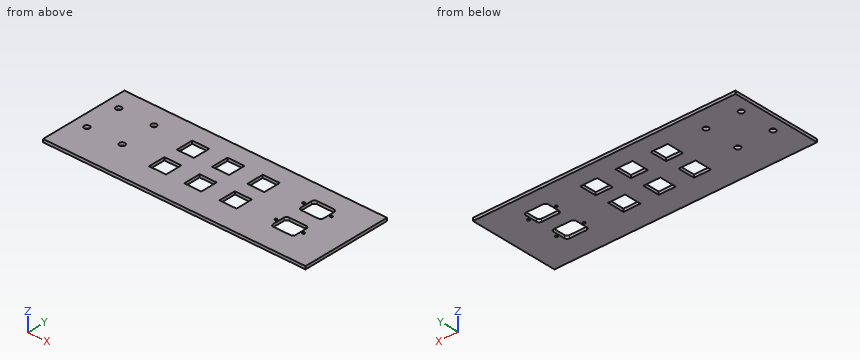
```python
from build123d import *

# Parameters (mm, degrees)
SKETCH1_W               = 378.46
SKETCH1_H               = 129.9972
BOSS_EXTRUDE1_DEPTH     = 4.191
F_3_8_16_TAPPED_HOLE1_D = 7.9375
CUT_EXTRUDE1_REACH      = 402.186
SKETCH5_W               = 24.5
SKETCH5_H               = 24.5
CUT_EXTRUDE2_REACH      = 402.186
SKETCH7_R               = 1.75


with BuildPart() as part:
    # Sketch1 → Boss-Extrude1 (new body)
    with BuildSketch(Plane.XY):
        with Locations((189.23, 64.9986)):
            Rectangle(SKETCH1_W, SKETCH1_H)
    extrude(amount=BOSS_EXTRUDE1_DEPTH)

    # 3/8-16 Tapped Hole1 (through all)
    with Locations(Plane.XY.offset(4.191)):
        with Locations((19.05, 99.8347), (69.85, 99.8347), (69.85, 49.0347), (19.05, 49.0347)):
            Hole(F_3_8_16_TAPPED_HOLE1_D / 2)

    # Sketch5 → Cut-Extrude1 (cut, up to next)
    with BuildSketch(Plane.XY.offset(4.191), mode=Mode.PRIVATE) as cut_extrude1_sk1:
        with Locations((132.9, 92.3472)):
            Rectangle(SKETCH5_W, SKETCH5_H)
    cut_extrude1_tool1 = extrude(cut_extrude1_sk1.sketch, amount=-CUT_EXTRUDE1_REACH, mode=Mode.PRIVATE) & part.part
    # Sketch5 → Cut-Extrude1 (cut, up to next)
    with BuildSketch(Plane.XY.offset(4.191), mode=Mode.PRIVATE) as cut_extrude1_sk2:
        with Locations((183.7, 92.3472)):
            Rectangle(SKETCH5_W, SKETCH5_H)
    cut_extrude1_tool2 = extrude(cut_extrude1_sk2.sketch, amount=-CUT_EXTRUDE1_REACH, mode=Mode.PRIVATE) & part.part
    # Sketch5 → Cut-Extrude1 (cut, up to next)
    with BuildSketch(Plane.XY.offset(4.191), mode=Mode.PRIVATE) as cut_extrude1_sk3:
        with Locations((234.5, 92.3472)):
            Rectangle(SKETCH5_W, SKETCH5_H)
    cut_extrude1_tool3 = extrude(cut_extrude1_sk3.sketch, amount=-CUT_EXTRUDE1_REACH, mode=Mode.PRIVATE) & part.part
    # Sketch5 → Cut-Extrude1 (cut, up to next)
    with BuildSketch(Plane.XY.offset(4.191), mode=Mode.PRIVATE) as cut_extrude1_sk4:
        with Locations((183.7, 47.8972)):
            Rectangle(SKETCH5_W, SKETCH5_H)
    cut_extrude1_tool4 = extrude(cut_extrude1_sk4.sketch, amount=-CUT_EXTRUDE1_REACH, mode=Mode.PRIVATE) & part.part
    # Sketch5 → Cut-Extrude1 (cut, up to next)
    with BuildSketch(Plane.XY.offset(4.191), mode=Mode.PRIVATE) as cut_extrude1_sk5:
        with Locations((234.5, 47.8972)):
            Rectangle(SKETCH5_W, SKETCH5_H)
    cut_extrude1_tool5 = extrude(cut_extrude1_sk5.sketch, amount=-CUT_EXTRUDE1_REACH, mode=Mode.PRIVATE) & part.part
    # Sketch5 → Cut-Extrude1 (cut, up to next)
    with BuildSketch(Plane.XY.offset(4.191), mode=Mode.PRIVATE) as cut_extrude1_sk6:
        with Locations((132.9, 47.8972)):
            Rectangle(SKETCH5_W, SKETCH5_H)
    cut_extrude1_tool6 = extrude(cut_extrude1_sk6.sketch, amount=-CUT_EXTRUDE1_REACH, mode=Mode.PRIVATE) & part.part
    add(cut_extrude1_tool1.solids().sort_by_distance((132.9, 92.3472, 4.191))[0], mode=Mode.SUBTRACT)
    add(cut_extrude1_tool2.solids().sort_by_distance((183.7, 92.3472, 4.191))[0], mode=Mode.SUBTRACT)
    add(cut_extrude1_tool3.solids().sort_by_distance((234.5, 92.3472, 4.191))[0], mode=Mode.SUBTRACT)
    add(cut_extrude1_tool4.solids().sort_by_distance((183.7, 47.8972, 4.191))[0], mode=Mode.SUBTRACT)
    add(cut_extrude1_tool5.solids().sort_by_distance((234.5, 47.8972, 4.191))[0], mode=Mode.SUBTRACT)
    add(cut_extrude1_tool6.solids().sort_by_distance((132.9, 47.8972, 4.191))[0], mode=Mode.SUBTRACT)

    # Sketch7 → Cut-Extrude2 (cut, up to next)
    with BuildSketch(Plane.XY.offset(4.191), mode=Mode.PRIVATE) as cut_extrude2_sk1:
        with Locations((292.657, 92.0972)):
            Circle(SKETCH7_R)
    cut_extrude2_tool1 = extrude(cut_extrude2_sk1.sketch, amount=-CUT_EXTRUDE2_REACH, mode=Mode.PRIVATE) & part.part
    # Sketch7 → Cut-Extrude2 (cut, up to next)
    with BuildSketch(Plane.XY.offset(4.191), mode=Mode.PRIVATE) as cut_extrude2_sk2:
        with Locations((332.657, 92.0972)):
            Circle(SKETCH7_R)
    cut_extrude2_tool2 = extrude(cut_extrude2_sk2.sketch, amount=-CUT_EXTRUDE2_REACH, mode=Mode.PRIVATE) & part.part
    # Sketch7 → Cut-Extrude2 (cut, up to next)
    with BuildSketch(Plane.XY.offset(4.191), mode=Mode.PRIVATE) as cut_extrude2_sk3:
        with Locations((332.657, 47.6472)):
            Circle(SKETCH7_R)
    cut_extrude2_tool3 = extrude(cut_extrude2_sk3.sketch, amount=-CUT_EXTRUDE2_REACH, mode=Mode.PRIVATE) & part.part
    # Sketch7 → Cut-Extrude2 (cut, up to next)
    with BuildSketch(Plane.XY.offset(4.191), mode=Mode.PRIVATE) as cut_extrude2_sk4:
        with Locations((292.657, 47.6472)):
            Circle(SKETCH7_R)
    cut_extrude2_tool4 = extrude(cut_extrude2_sk4.sketch, amount=-CUT_EXTRUDE2_REACH, mode=Mode.PRIVATE) & part.part
    # Sketch7 → Cut-Extrude2 (cut, up to next)
    with BuildSketch(Plane.XY.offset(4.191), mode=Mode.PRIVATE) as cut_extrude2_sk5:
        with BuildLine():
            Line((300.407, 60.1472), (324.907, 60.1472))
            ThreePointArc((324.907, 60.1472), (327.735427125, 58.975627125), (328.907, 56.1472))
            Line((328.907, 56.1472), (328.907, 39.1472))
            ThreePointArc((328.907, 39.1472), (327.735427125, 36.318772875), (324.907, 35.1472))
            Line((324.907, 35.1472), (300.407, 35.1472))
            ThreePointArc((300.407, 35.1472), (297.578572875, 36.318772875), (296.407, 39.1472))
            Line((296.407, 39.1472), (296.407, 56.1472))
            ThreePointArc((296.407, 56.1472), (297.578572875, 58.975627125), (300.407, 60.1472))
        make_face()
    cut_extrude2_tool5 = extrude(cut_extrude2_sk5.sketch, amount=-CUT_EXTRUDE2_REACH, mode=Mode.PRIVATE) & part.part
    # Sketch7 → Cut-Extrude2 (cut, up to next)
    with BuildSketch(Plane.XY.offset(4.191), mode=Mode.PRIVATE) as cut_extrude2_sk6:
        with BuildLine():
            Line((300.407, 104.5972), (324.907, 104.5972))
            ThreePointArc((324.907, 104.5972), (327.735427125, 103.425627125), (328.907, 100.5972))
            Line((328.907, 100.5972), (328.907, 83.5972))
            ThreePointArc((328.907, 83.5972), (327.735427125, 80.768772875), (324.907, 79.5972))
            Line((324.907, 79.5972), (300.407, 79.5972))
            ThreePointArc((300.407, 79.5972), (297.578572875, 80.768772875), (296.407, 83.5972))
            Line((296.407, 83.5972), (296.407, 100.5972))
            ThreePointArc((296.407, 100.5972), (297.578572875, 103.425627125), (300.407, 104.5972))
        make_face()
    cut_extrude2_tool6 = extrude(cut_extrude2_sk6.sketch, amount=-CUT_EXTRUDE2_REACH, mode=Mode.PRIVATE) & part.part
    add(cut_extrude2_tool1.solids().sort_by_distance((292.657, 92.0972, 4.191))[0], mode=Mode.SUBTRACT)
    add(cut_extrude2_tool2.solids().sort_by_distance((332.657, 92.0972, 4.191))[0], mode=Mode.SUBTRACT)
    add(cut_extrude2_tool3.solids().sort_by_distance((332.657, 47.6472, 4.191))[0], mode=Mode.SUBTRACT)
    add(cut_extrude2_tool4.solids().sort_by_distance((292.657, 47.6472, 4.191))[0], mode=Mode.SUBTRACT)
    add(cut_extrude2_tool5.solids().sort_by_distance((312.657, 47.6472, 4.191))[0], mode=Mode.SUBTRACT)
    add(cut_extrude2_tool6.solids().sort_by_distance((312.657, 92.0972, 4.191))[0], mode=Mode.SUBTRACT)


solid = part.part
```
Read the model definition and answer for the solid it produces. Units are mm, in the model's axes. Give positions to 0.01 mm unless a question says otherwise; leave off trailing zeros. Loops run counter-clockwise (first coordinate to the right, second up) from the corner with the lowest first, then second, coordinate; pieces in that order, holes last.
Item 1: The part is cut by section B-B (x = 140). Write down the section's boundary in (y, z), and give its area (3 significant figures).
Item 2: The part is cut by section C-C (z = 2.7). Give the number of separate pieces and of enclosed holes in the cut face, and give its area (3 significant figures).
Item 3: The part is cut by section A-A (x = 69.85). Write down the section's boundary in (y, z).
Item 4: Each of these flat-tipped pins is pushed along its axis until it touches: pin 1 Ø12.5 at (x, y) = (69.85, 49.03) entering from +Z; pin 2 Ø2 at (x, y) = (313.5, 102.5) entering from +Z. Where does it stop, or does it pass through?
Item 5: Find the intervals of material crossed by line 1 along Y through (x, z) = (245, 3); line 2 along X through (y, z) = (83, 2.9); line 3 along X through (y, z) = (42, 1.7), in increasing order.
Taken from the geometry:
1. outline: (0, 0) - (35.65, 0) - (35.65, 4.19) - (0, 4.19) - close; (60.15, 0) - (80.1, 0) - (80.1, 4.19) - (60.15, 4.19) - close; (104.6, 0) - (130, 0) - (130, 4.19) - (104.6, 4.19) - close
1. area: 339 mm2
2. separate pieces: 1
2. enclosed holes: 16
2. area: 43,800 mm2
3. outline: (0, 0) - (45.07, 0) - (45.07, 4.19) - (0, 4.19) - close; (53, 0) - (95.87, 0) - (95.87, 4.19) - (53, 4.19) - close; (103.8, 0) - (130, 0) - (130, 4.19) - (103.8, 4.19) - close
4. pin 1: stops at z = 4.19
4. pin 2: passes through
5. line 1: y = 0 to 35.65, 60.15 to 80.1, 104.6 to 130
5. line 2: x = 0 to 120.65, 145.15 to 171.45, 195.95 to 222.25, 246.75 to 296.45, 328.86 to 378.46
5. line 3: x = 0 to 120.65, 145.15 to 171.45, 195.95 to 222.25, 246.75 to 296.41, 328.91 to 378.46
